Can you work these out from the model? Positions are in its coordinate system, mm. A direction names the side the tool comes from. Coordinates: 2 decimals unless noted, no trailing zeros. Order: outer loops, then holes, each group sorted by start corner. A loop starts at its lowest first (then second) coordinate and runs counter-clockwise, first axis right, second up. Notation, with made-up numbers: (-9, 66.25) -> (33, 66.25) arc R16 cw to (33, 78.25) -> close; hole circle Ø1 at (2.5, 40). An arc over 180 degrees is marked (long way). Answer in a Markdown table with one row per item. Add a question column.
1. If I drill on line 1 along Z through (x, y) = (13, -9.5); line 2 along Y through (x, z) = (-4.5, -0.25); line 3 along Y through (x, z) = (-12, 0.75), over which ranges is the centre line in solid material (lowest first)? Write a range as [from, to].
2. Will these pins go through, and if not, where does the flat tip stop? pin 1 (1.5 mm diameter, centred on x = -13, z = 1.5, fed in from +Y); pin 2 (8 mm diameter, centred on x = -1, y = -12.5, fed in from -Z); pin 3 (3 mm diameter, centred on x = 0.5, z = 1.5, fed in from +Y).
3. On a 3-axis mill with a long thin cutter (end or side, diameter ignored), from which of +Z, -Z, +X, -X, +Y, -Y can I reach the whole of each face in a straight line? I mean faces 1 (the face through (8, 0, 0)), 2 (the face through (0, 0, -4.826)). Say none if no direction works.
4. Imagine slicing it at A-A on x = 0. Write out the boundary of the cut face in (y, z), plus the area to 3 significant figures.
5. Imagine slicing it at C-C on z = -2.5. Write out the boundary of the cut face in (x, y).
6. Imagine slicing it at D-D on z = 0.75. Write out the boundary of the cut face in (x, y), plus the area to 3 significant figures.
from build123d import *

# Parameters (mm, degrees)
F0_R     = 2.25
F1_DEPTH = 2.54
F0_R_2   = 19.05
F2_DEPTH = 2.54
F3_R     = 7.47
F4_DEPTH = 4.826


with BuildPart() as f1:
    # F0 (on Top) → F1 (new body)
    with BuildSketch(Plane.XY):
        Circle(F0_R)
    extrude(amount=F1_DEPTH)

    # F0 (on Top) → F2 (join)
    with BuildSketch(Plane.XY):
        Circle(F0_R_2)
        Circle(F0_R, mode=Mode.SUBTRACT)
    extrude(amount=F2_DEPTH)

    # F3 (on face) → F4 (join)
    with BuildSketch(Plane(origin=(0, 0, 0), x_dir=(1, 0, 0), z_dir=(0, 0, -1))):
        Circle(F3_R)
    extrude(amount=F4_DEPTH)


solid = f1.part
Answers follow:
| question | item | result |
|---|---|---|
| 1 | line 1 | z = [0, 2.54] |
| 1 | line 2 | y = [-5.96, 5.96] |
| 1 | line 3 | y = [-14.8, 14.8] |
| 2 | pin 1 | stops at y = 14.59 |
| 2 | pin 2 | stops at z = 0 |
| 2 | pin 3 | stops at y = 19.05 |
| 3 | face 1 | -Z |
| 3 | face 2 | -Z, +X, -X, +Y, -Y |
| 4 | outline | (-19.05, 0) -> (-7.47, 0) -> (-7.47, -4.83) -> (7.47, -4.83) -> (7.47, 0) -> (19.05, 0) -> (19.05, 2.54) -> (-19.05, 2.54) -> close |
| 4 | area | 169 mm² |
| 5 | outline | circle Ø14.94 at (0, 0) |
| 6 | outline | circle Ø38.1 at (0, 0) |
| 6 | area | 1,140 mm² |
